The model under review builds one solid part; all positions refer to its coordinate system, in mm. Face numbers are marked on the shaded views. A direction names the side the tool comes from. Coordinates: 2 decimals unless noted, no trailing zeros. Write each loop counter-clockwise with the first axis right and the second up, starting at its lowest first coordinate (ties: lowest second). Pieces come first, ordered by that corner, then holes. Notation, with made-up numbers: (49.5, 54.5) - (66.5, 54.5) arc R24 ccw to (66.5, 86.5) - close; hole circle Ø11 at (15.5, 76). An arc over 180 degrees is marked (long way). Put each result on its own line as item: value. Start each with the question number.
Item 1: Consider section B-B on z = 2. Give the boundary of the cut face in (x, y), then the cut area to 3 significant figures.
Item 2: Consider section A-A on y = 9.25. Give the boundary of the cut face in (x, z).
Item 3: Consider section C-C on x = -15.5. State how many separate pieces and enclosed holes the cut face has, then the cut area to 3 significant figures.
Item 4: For pin 1 (1 mm diameter, centred on x = -23.5, y = 16.5, fed in from -Z); pin 2 (2 mm diameter, centred on x = -26, z = -12.5, fed in from -Y); pin 3 (0.5 mm diameter, centred on y = 13, z = -15, fed in from +X); pin 4 (5 mm diameter, centred on x = -17.5, z = 23, fed in from +Y), all flat-tipped, find the tip position at first contact; note any pin that passes through.
Item 5: To check wall thickness, follow L1, parallel to Y at x = -16.75, z = 15.5; L2, parallel to Z at x = -23.5, y = 4.5; L3, parallel to Y at x = -17.25, z = -22. State the ranges of each line that lie inside material, in increasing order. Write a range as [from, to].
Item 6: Mouldability with a two-part tool opening along Z and no side actions: class the marked faces 1, 2 and 3 as pulls with the +Z half, pulls with the -Z half, needs draft (parallel to the pull), parting line crosses it, or undercut.
Item 7: Machinability: for the marked faces 4, 5, 6, 7 and 8, which of the approach directions +Z, -Z, +X, -X, +Y, -Y give a long, thin tool a straight path to every point of the face, cutting with its end or side? Answer none if there is none.
```python
from build123d import *

# Parameters (mm, degrees)
SKETCH3_R           = 1.2
BOSS_EXTRUDE1_DEPTH = 25
SKETCH5_W           = 28
SKETCH5_H           = 22
CUT_EXTRUDE1_DEPTH  = 43.03807243
CUT_EXTRUDE2_DEPTH  = 22
SKETCH8_W           = 3
SKETCH8_H           = 3
BOSS_EXTRUDE2_DEPTH = 3
SKETCH9_W           = 11.23999152
SKETCH9_H           = 22
CUT_EXTRUDE3_DEPTH  = 47.686959369
SKETCH10_W          = 11.23999152
SKETCH10_H          = 13
CUT_EXTRUDE4_DEPTH  = 61.429893223
FILLET1_START       = -17
FILLET1_DEPTH       = 3
FILLET1_START_2     = 14
FILLET1_2_DEPTH     = 3
FILLET1_START_3     = 22
FILLET1_3_DEPTH     = 3
FILLET1_START_4     = -30.6499947
FILLET1_4_DEPTH     = 61.2999894
FILLET1_START_5     = 19.56628
FILLET1_5_DEPTH     = 6.43372
FILLET2_R           = 1
FILLET3_R           = 1
FILLET4_R           = 1.5


with BuildPart() as part:
    # Sketch3 → Boss-Extrude1 (new body)
    with BuildSketch(Plane(origin=(0, 0, 0), x_dir=(1, 0, 0), z_dir=(0, 1, 0))):
        Polygon((-13.26000848, 30.6499947), (-27.5, 21.75), (-27.5, -21.75), (-13.26000848, -30.6499947), align=None)
        with Locations(Location((-18.538627315, 21.642919742, 0), (0, 0, 270))):
            Circle(SKETCH3_R, mode=Mode.SUBTRACT)
        with Locations(Location((-16.127132138, 25.803411421, 0), (0, 0, 270))):
            Circle(SKETCH3_R, mode=Mode.SUBTRACT)
        with Locations(Location((-18.538627315, -21.642919742, 0), (0, 0, 270))):
            Circle(SKETCH3_R, mode=Mode.SUBTRACT)
        with Locations(Location((-16.127132138, -25.803411421, 0), (0, 0, 270))):
            Circle(SKETCH3_R, mode=Mode.SUBTRACT)
    extrude(amount=BOSS_EXTRUDE1_DEPTH)

    # Sketch5 → Cut-Extrude1 (cut, through all)
    with BuildSketch(Plane(origin=(-13.26000848, 0, 0), x_dir=(0, 0, -1), z_dir=(1, 0, 0))):
        with Locations((0, 11)):
            Rectangle(SKETCH5_W, SKETCH5_H)
    extrude(amount=-CUT_EXTRUDE1_DEPTH, mode=Mode.SUBTRACT)

    # Sketch6 → Cut-Extrude2 (cut)
    with BuildSketch(Plane(origin=(0, 25, 0), x_dir=(1, 0, 0), z_dir=(0, 1, 0))):
        Polygon((-13.26000848, -30.6499947), (-27.5, -21.75), (-27.5, -17), (-13.26000848, -17), align=None)
        Polygon((-27.5, 17), (-27.5, 21.75), (-13.26000848, 30.6499947), (-13.26000848, 17), align=None)
    extrude(amount=-CUT_EXTRUDE2_DEPTH, mode=Mode.SUBTRACT)

    # Sketch8 → Boss-Extrude2 (add)
    with BuildSketch(Plane.XZ.offset(-22)):
        with Locations((-26, -12.5)):
            Rectangle(SKETCH8_W, SKETCH8_H)
        with Locations((-26, 12.5)):
            Rectangle(SKETCH8_W, SKETCH8_H)
    extrude(amount=BOSS_EXTRUDE2_DEPTH)

    # Sketch9 → Cut-Extrude3 (cut, through all)
    with BuildSketch(Plane.XZ.offset(-22)):
        with Locations((-18.88000424, 0)):
            Rectangle(SKETCH9_W, SKETCH9_H)
    extrude(amount=-CUT_EXTRUDE3_DEPTH, mode=Mode.SUBTRACT)

    # Sketch10 → Cut-Extrude4 (cut, through all)
    with BuildSketch(Plane(origin=(0, 0, -17), x_dir=(-1, 0, 0), z_dir=(0, 0, -1))):
        with Locations((18.88000424, 12.5)):
            Rectangle(SKETCH10_W, SKETCH10_H)
    extrude(amount=-CUT_EXTRUDE4_DEPTH, mode=Mode.SUBTRACT)

    # Fillet1: read off the stored shape, not the designer's step
    # Fillet1 outline → Fillet1 (add)
    with BuildSketch(Plane.XY.offset(FILLET1_START)):
        with BuildLine():
            Line((-24.5, 19), (-24.5, 17.5))
            ThreePointArc((-24.5, 17.5), (-24.060660172, 18.560660172), (-23, 19))
            Line((-23, 19), (-24.5, 19))
        make_face()
        with BuildLine():
            Line((-24.5, 6), (-23, 6))
            ThreePointArc((-23, 6), (-24.060660172, 6.439339828), (-24.5, 7.5))
            Line((-24.5, 7.5), (-24.5, 6))
        make_face()
    extrude(amount=FILLET1_DEPTH)

    # Fillet1 2 outline → Fillet1 2 (add)
    with BuildSketch(Plane.XY.offset(FILLET1_START_2)):
        with BuildLine():
            Line((-24.5, 19), (-24.5, 17.5))
            ThreePointArc((-24.5, 17.5), (-24.060660172, 18.560660172), (-23, 19))
            Line((-23, 19), (-24.5, 19))
        make_face()
        with BuildLine():
            Line((-24.5, 6), (-23, 6))
            ThreePointArc((-23, 6), (-24.060660172, 6.439339828), (-24.5, 7.5))
            Line((-24.5, 7.5), (-24.5, 6))
        make_face()
    extrude(amount=FILLET1_2_DEPTH)

    # Fillet1 3 outline → Fillet1 3 (add)
    with BuildSketch(Plane(origin=(0, 0, 0), x_dir=(1, 0, 0), z_dir=(0, 1, 0)).offset(FILLET1_START_3)):
        with BuildLine():
            ThreePointArc((-23, -11), (-24.060660172, -10.560660172), (-24.5, -9.5))
            Line((-24.5, -9.5), (-24.5, -11))
            Line((-24.5, -11), (-23, -11))
        make_face()
        with BuildLine():
            ThreePointArc((-24.5, 9.5), (-24.060660172, 10.560660172), (-23, 11))
            Line((-23, 11), (-24.5, 11))
            Line((-24.5, 11), (-24.5, 9.5))
        make_face()
    extrude(amount=FILLET1_3_DEPTH)

    # Fillet1 4 outline → Fillet1 4 (cut)
    with BuildSketch(Plane.XY.offset(FILLET1_START_4)):
        with BuildLine():
            Line((-13.26000848, 6), (-14.76000848, 6))
            ThreePointArc((-14.76000848, 6), (-13.699348308, 5.560660172), (-13.26000848, 4.5))
            Line((-13.26000848, 4.5), (-13.26000848, 6))
        make_face()
        with BuildLine():
            ThreePointArc((-13.26000848, 20.5), (-13.699348308, 19.439339828), (-14.76000848, 19))
            Line((-14.76000848, 19), (-13.26000848, 19))
            Line((-13.26000848, 19), (-13.26000848, 20.5))
        make_face()
    extrude(amount=FILLET1_4_DEPTH, mode=Mode.SUBTRACT)

    # Fillet1 5 outline → Fillet1 5 (cut)
    with BuildSketch(Plane(origin=(0, 0, 0), x_dir=(1, 0, 0), z_dir=(0, 1, 0)).offset(FILLET1_START_5)):
        with BuildLine():
            Line((-13.26000848, 11), (-13.26000848, 12.5))
            ThreePointArc((-13.26000848, 12.5), (-13.699348308, 11.439339828), (-14.76000848, 11))
            Line((-14.76000848, 11), (-13.26000848, 11))
        make_face()
        with BuildLine():
            Line((-13.26000848, -11), (-14.76000848, -11))
            ThreePointArc((-14.76000848, -11), (-13.699348308, -11.439339828), (-13.26000848, -12.5))
            Line((-13.26000848, -12.5), (-13.26000848, -11))
        make_face()
    extrude(amount=FILLET1_5_DEPTH, mode=Mode.SUBTRACT)

    # Fillet2
    fillet2_edges = [part.edges().sort_by_distance(p)[0] for p in [
        (-24.5, 22, -12.5),
        (-24.5, 20.5, -14),
        (-26, 22, -11),
        (-24.5, 20.5, -11),
        (-26, 19, -14),
        (-24.5, 19, -12.5),
        (-24.5, 20.5, 14),
        (-26, 22, 11),
        (-24.5, 22, 12.5),
        (-24.5, 20.5, 11),
        (-26, 19, 14),
        (-24.5, 19, 12.5),
    ]]
    fillet(fillet2_edges, radius=FILLET2_R)

    # Fillet3
    # the kernel refuses this fillet: 1 mm, written as the material it adds along each edge
    with BuildSketch(Plane(origin=(-23.5, 21, 13), x_dir=(0, 1, 0), z_dir=(0, 0, 1))) as fillet3_piece_1_section:
        Polygon((0, 0), (FILLET3_R, 0), (FILLET3_R, FILLET3_R), (0, FILLET3_R), align=None)
    fillet3_piece_1 = extrude(amount=FILLET3_R, mode=Mode.PRIVATE)
    fillet3_piece_1 = fillet3_piece_1 - Plane(origin=(-23.5, 21, 13), x_dir=(0.7071067811865475, -0.7071067811865475, 0), z_dir=(0, 0, 1)) * Sphere(FILLET3_R, mode=Mode.PRIVATE)
    add(fillet3_piece_1)
    with BuildSketch(Plane(origin=(-23.5, 21, -13), x_dir=(0, 0, -1), z_dir=(0, 1, 0))) as fillet3_piece_2_section:
        Polygon((0, 0), (FILLET3_R, 0), (FILLET3_R, FILLET3_R), (0, FILLET3_R), align=None)
    fillet3_piece_2 = extrude(amount=FILLET3_R, mode=Mode.PRIVATE)
    fillet3_piece_2 = fillet3_piece_2 - Plane(origin=(-23.5, 21, -13), x_dir=(0.7071067811865691, 0, 0.707106781186526), z_dir=(0, 1, 0)) * Sphere(FILLET3_R, mode=Mode.PRIVATE)
    add(fillet3_piece_2)
    with BuildSketch(Plane(origin=(-13.26000848, 22, 14), x_dir=(0, -1, 0), z_dir=(-1, 0, 0)), Plane(origin=(-13.26000848, 22, -14), x_dir=(0, 0, 1), z_dir=(-1, 0, 0))) as fillet3_piece_3:
        with BuildLine():
            CenterArc((FILLET3_R, -FILLET3_R), FILLET3_R, 90, 90)
            Line((0, -FILLET3_R), (0, 0))
            Line((0, 0), (FILLET3_R, 0))
        make_face()
    extrude(amount=10.23999152)
    # the kernel refuses this fillet: 1 mm, written as the material it takes off along each edge
    with BuildSketch(Plane(origin=(-10.76000848, 0, 14), x_dir=(0, 1, 0), z_dir=(-1, 0, 0)), Plane(origin=(-10.76000848, 0, -14), x_dir=(0, 0, -1), z_dir=(-1, 0, 0))) as fillet3_2_piece_1:
        with BuildLine():
            CenterArc((FILLET3_R, -FILLET3_R), FILLET3_R, 90, 90)
            Line((0, -FILLET3_R), (0, 0))
            Line((0, 0), (FILLET3_R, 0))
        make_face()
    extrude(amount=19.23999152, mode=Mode.SUBTRACT)

    # Fillet4
    fillet4_edges = [part.edges().sort_by_distance(p)[0] for p in [
        (-13.26000848, 3, -23.82499735),
        (-13.26000848, 3, 23.82499735),
        (-13.699348308, 5.560660172, -17),
        (-18.88000424, 6, -17),
        (-24.060660172, 6.439339828, -17),
        (-24.5, 12.5, -17),
        (-24.060660172, 18.560660172, -17),
        (-18.88000424, 19, -17),
        (-13.699348308, 19.439339828, -17),
        (-13.26000848, 25, -14.75),
        (-13.699348308, 25, -11.439339828),
        (-18.88000424, 25, -11),
        (-24.060660172, 25, -10.560660172),
        (-24.5, 25, 0),
        (-24.060660172, 25, 10.560660172),
        (-18.88000424, 25, 11),
        (-13.699348308, 25, 11.439339828),
        (-13.699348308, 5.560660172, 17),
        (-18.88000424, 6, 17),
        (-24.060660172, 6.439339828, 17),
        (-24.5, 12.5, 17),
        (-24.060660172, 18.560660172, 17),
        (-18.88000424, 19, 17),
        (-13.699348308, 19.439339828, 17),
        (-20.38000424, 3, 17),
        (-20.38000424, 3, -17),
        (-13.26000848, 22.75, -17),
        (-13.26000848, 25, 14.75),
        (-13.26000848, 22.75, 17),
        (-20.38000424, 25, 17),
        (-20.38000424, 25, -17),
    ]]
    fillet(fillet4_edges, radius=FILLET4_R - 0.0001)  # a hair under: the kernel refuses the full size


solid = part.part
```
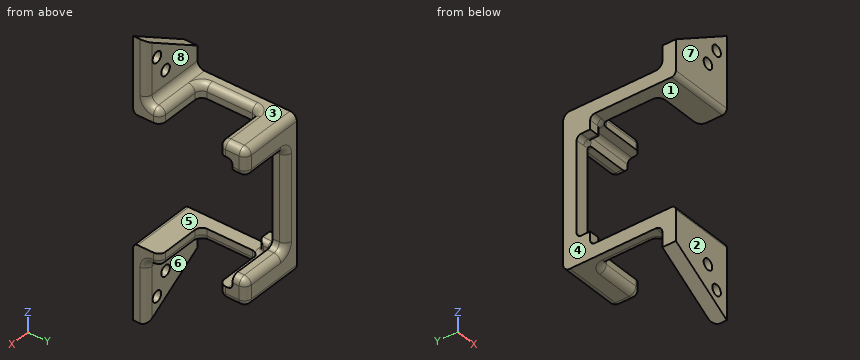
Report:
1. outline: (-27.5, 22) - (-24.5, 22) - (-24.5, 23.5) arc R1.5 ccw to (-26, 25) - (-27.5, 25) - close
1. area: 8.52 mm²
2. outline: (-27.5, -17) - (-26, -17) arc R1.5 ccw to (-24.5, -15.5) - (-24.5, -14) - (-27.5, -14) - close; (-27.5, 14) - (-24.5, 14) - (-24.5, 15.5) arc R1.5 ccw to (-26, 17) - (-27.5, 17) - close
3. separate pieces: 6
3. enclosed holes: 0
3. area: 148 mm²
4. pin 1: through
4. pin 2: y = 18.87
4. pin 3: x = -24.5
4. pin 4: y = 3
5. L1: [0, 6], [19, 25]
5. L2: [-17, -14], [14, 17]
5. L3: [0, 3]
6. face 1: undercut
6. face 2: needs draft
6. face 3: pulls with the +Z half
7. face 4: +Z, -Z, -X, +Y, -Y
7. face 5: +X, -Y
7. face 6: -Z, +X, -X, +Y
7. face 7: +Z, -Z, +X, -X, -Y
7. face 8: +Z, +X, -X, +Y
